The model under review builds one solid part; all positions refer to its coordinate system, in mm. A direction names the side the tool comes from. Round coordinates to 2 decimals unless told otherwise and drop trailing zeros. Order: outer loops, then holes, each group sorted by start corner. A loop starts at its lowest first (then second) coordinate and runs counter-clockwise, first axis right, second up. Notation, with made-up numbers: (-3, 77) - (21, 77) arc R35 ccw to (21, 116) - close; hole circle Ø4 at (-20, -24.75). An arc over 180 degrees is marked (long way). One line per question, with ' | ' between items. Start each with the question number.
Item 1: Draft analysis for pull direction X (two halves, no side actions). For faces 3 (the face through (-22, 1, 0)), 4 (the face through (-24, 0, 0)), 5 (the face through (0, -8, -12.5)), 6 (the face through (22, 1, 0)), state which applies: +X half, -X half, draft (parallel to the pull), parting line (faces both ways), or undercut.
Item 2: Add section A-A on y = 3.5. State the section outline as (x, z) points, and give its area (3 significant figures).
Item 3: Insertion check: pin 1 Ø7.5 at (x, z) = (-1.5, 6) entering from +Y. The pin has a flat end and moves straight along its axis. Give the tip position at first contact, or say it passes through.
Item 4: For L1, parallel to X at y = -4.5, z = -7.5; L2, parallel to Y at x = -3, z = 8.75, list the stretches that pass through material, from the lowest coordinate up. Write a range as [from, to].
Item 5: Tool access review of faces 1 (the face through (0, -6.5, 0)), 2 (the face through (-23, 8.5, 0)): name each direction out of +Z, -Z, +X, -X, +Y, -Y from which nothing blocks a thin tool from reaching the whole face with its end or side.
Item 6: Add section C-C on x = -10. State the section outline as (y, z) points, and give its area (3 significant figures).
Item 7: Add section B-B on z = 1.25. State the section outline as (x, y) points.
from build123d import *

# Parameters (mm, degrees)
ESBO_O1_W                = 48
ESBO_O1_H                = 25
RESSALTO_EXTRUS_O1_DEPTH = 8.5
CASCA1_T                 = -2


with BuildPart() as part:
    # Esboço1 → Ressalto-extrusão1 (new, symmetric)
    with BuildSketch(Plane(origin=(0, 0, 0), x_dir=(1, 0, 0), z_dir=(0, 1, 0))):
        Rectangle(ESBO_O1_W, ESBO_O1_H)
    extrude(amount=RESSALTO_EXTRUS_O1_DEPTH, both=True)

    # Casca1
    casca1_openings = [part.faces().sort_by_distance(p)[0] for p in [
        (0, 8.5, 0),
        (0, 0, 12.5),
        (0, 0, -12.5),
    ]]
    offset(amount=CASCA1_T, openings=casca1_openings, kind=Kind.INTERSECTION)


solid = part.part
Determined:
1) face 3: undercut | face 4: -X half | face 5: draft | face 6: undercut
2) outline: (-24, -12.5) - (-22, -12.5) - (-22, 12.5) - (-24, 12.5) - close; (22, -12.5) - (24, -12.5) - (24, 12.5) - (22, 12.5) - close | area: 100 mm2
3) pin 1: y = -6.5
4) L1: [-24, -22], [22, 24] | L2: [-8.5, -6.5]
5) face 1: +Z, -Z, +Y | face 2: +Z, -Z, +X, -X, +Y
6) outline: (-8.5, -12.5) - (-6.5, -12.5) - (-6.5, 12.5) - (-8.5, 12.5) - close | area: 50.0 mm2
7) outline: (-24, -8.5) - (24, -8.5) - (24, 8.5) - (22, 8.5) - (22, -6.5) - (-22, -6.5) - (-22, 8.5) - (-24, 8.5) - close
